```python
from build123d import *

# Parameters (mm, degrees)
F0_W     = 55
F0_H     = 30
F1_DEPTH = 30
F2_W     = 25.139422
F2_H     = 16
F3_DEPTH = 67.1
F4_R     = 7.5
F5_DEPTH = 5
F6_DEPTH = 5


with BuildPart() as f1:
    # F0 (on Top) → F1 (new body)
    with BuildSketch(Plane.XY):
        Rectangle(F0_W, F0_H)
    extrude(amount=F1_DEPTH)

    # F2 (on Top) → F3 (cut)
    with BuildSketch(Plane.XY):
        with Locations((-15.522837, 8)):
            Rectangle(F2_W, F2_H)
    extrude(amount=F3_DEPTH, mode=Mode.SUBTRACT)

    # F4 (on Top) → F5 (cut)
    with BuildSketch(Plane.XY):
        with Locations((17.489556, -15.456908)):
            Circle(F4_R)
    extrude(amount=F5_DEPTH, mode=Mode.SUBTRACT)

    # F4 (on Top) → F6 (cut)
    with BuildSketch(Plane.XY):
        with Locations((-17.510444, -15.456908)):
            Circle(F4_R)
        with Locations((17.489556, -15.456908)):
            Circle(F4_R)
    extrude(amount=F6_DEPTH, mode=Mode.SUBTRACT)


solid = f1.part
```
Geometry: final body of the model. Coordinates: model frame, mm. A direction names the side the tool comes from. Give positions to 0.01 mm unless a question says otherwise; leave off trailing zeros. Order: outer loops, then holes, each group sorted by start corner. A loop starts at its lowest first (then second) coordinate and runs counter-clockwise, first axis right, second up. Notation, with made-up numbers: M -10.5,55 L 27.5,55 A29 ccw 27.5,86 Z; hole C 27.25,-22.5 d11. An arc over 180 degrees is marked long. Answer as CSV lines item,"result". Start each with the question number.
1) Cut plane D-D (z = 23). Output: boundary loops of the cut face in (x, y).
2) Line query: line 1 (X direction, y = -12, z = 3.25); line 2 (X direction, y = 14, z = 18.75); line 3 (X direction, y = -11.5, z = 4.75). Output: solid intervals per line, ascending. Write a range as from..to.
3) First-contact query: P1, Ø5.5, axis at x = 15.5, y = -11.5, coming from the -Z side. Flat tip, straight axial feed; report the tip coordinate or a pass-through.
4) Cut plane C-C (y = -12). Output: boundary loops of the cut face in (x, z), then the cut area to 3 significant figures.
5) Cut plane B-B (x = -11). Output: boundary loops of the cut face in (y, z).
6) Cut plane A-A (z = 4). Output: boundary loops of the cut face in (x, y).
7) Set-up query: faces 1 (the flat face through (-15, 0, 15)), 2 (the cylindrical face through (17.65, -7.96, 2.46)), 3 (the flat face through (0, -15, 18)). Return all of +Z, -Z, +X, -X, +Y, -Y with unobstructed straight access to the full face (end or side cutting, diameter ignored); none if empty.
8) Mould query, pull axis X, two halves, no side actions, for faces 4 (the cylindrical face through (-17.35, -7.96, 2.46)), 5 (the flat face through (-2.953, 7, 15)), 6 (the flat face through (12, 15, 15)). Classes: +X half, -X half, draft (parallel to the pull), parting line (faces both ways), or undercut.
Findings below:
1,outline,"M -27.5,-15 L 27.5,-15 L 27.5,15 L -2.95,15 L -2.95,0 L -27.5,0 Z"
2,line 1,"x = -27.5..-24.17, -10.85..10.83, 24.15..27.5"
2,line 2,"x = -2.95..27.5"
2,line 3,"x = -27.5..-23.88, -11.14..11.12, 23.86..27.5"
3,P1,"stops at z = 5"
4,outline,"M -27.5,0 L -24.17,0 L -24.17,5 L -10.85,5 L -10.85,0 L 10.83,0 L 10.83,5 L 24.15,5 L 24.15,0 L 27.5,0 L 27.5,30 L -27.5,30 Z"
4,area,"1,520 mm²"
5,outline,"M -15,5 L -11.73,5 L -11.73,0 L 0,0 L 0,30 L -15,30 Z"
6,outline,"M -27.5,-15 L -25,-15 A7.5 cw -10.02,-15 L 10,-15 A7.5 cw 24.98,-15 L 27.5,-15 L 27.5,15 L -2.95,15 L -2.95,0 L -27.5,0 Z"
7,face 1,"+Z, -Z, -X, +Y"
7,face 2,"-Z, -Y"
7,face 3,"+Z, -Z, +X, -X, -Y"
8,face 4,"undercut"
8,face 5,"-X half"
8,face 6,"draft"
